from build123d import *

# Parameters (mm, degrees)
SKETCH2_R           = 88.9
BOSS_EXTRUDE1_DEPTH = 3.175
SKETCH3_R           = 3.175
SKETCH3_W           = 50.8
SKETCH3_H           = 71.12
CUT_EXTRUDE1_DEPTH  = 3.175
SKETCH5_W           = 3
SKETCH5_H           = 3
SKETCH5_R           = 3.175
CUT_EXTRUDE2_DEPTH  = 126.763669734
FILLET1_R           = 22.86
SKETCH6_R           = 6.35
CUT_EXTRUDE3_DEPTH  = 126.763669734


with BuildPart() as part:
    # Sketch2 → Boss-Extrude1 (new body)
    with BuildSketch(Plane(origin=(0, 0, 0), x_dir=(1, 0, 0), z_dir=(0, 1, 0))):
        with Locations(Location((0, 0, 0), (0, 0, 270))):
            Circle(SKETCH2_R)
    extrude(amount=BOSS_EXTRUDE1_DEPTH)

    # Sketch3 → Cut-Extrude1 (cut)
    with BuildSketch(Plane(origin=(0, 3.175, 0), x_dir=(1, 0, 0), z_dir=(0, 1, 0))):
        with Locations(Location((65.549718535, -24.13, 0), (0, 0, 270))):
            Circle(SKETCH3_R)
        with Locations(Location((65.549718535, 24.13, 0), (0, 0, 270))):
            Circle(SKETCH3_R)
        with Locations(Location((-53.672052261, 44.702721462, 0), (0, 0, 270))):
            Circle(SKETCH3_R)
        with Locations(Location((-11.877666274, 68.832721462, 0), (0, 0, 270))):
            Circle(SKETCH3_R)
        with Locations(Location((-11.877666274, -68.832721462, 0), (0, 0, 270))):
            Circle(SKETCH3_R)
        with Locations(Location((-53.672052261, -44.702721462, 0), (0, 0, 270))):
            Circle(SKETCH3_R)
        with Locations((-63.5, 0)):
            Rectangle(SKETCH3_W, SKETCH3_H)
    extrude(amount=-CUT_EXTRUDE1_DEPTH, mode=Mode.SUBTRACT)

    # Sketch5 → Cut-Extrude2 (cut, through all)
    with BuildSketch(Plane(origin=(0, 3.175, 0), x_dir=(1, 0, 0), z_dir=(0, 1, 0))):
        with Locations((-36.6, 57.12)):
            Rectangle(SKETCH5_W, SKETCH5_H)
        with Locations((-28.98, 1.04)):
            Rectangle(SKETCH5_W, SKETCH5_H)
        with Locations(Location((61.9, 44.62, 0), (0, 0, 270))):
            Circle(SKETCH5_R)
        with Locations(Location((47.695, -21.96, 0), (0, 0, 270))):
            Circle(SKETCH5_R)
    extrude(amount=-CUT_EXTRUDE2_DEPTH, mode=Mode.SUBTRACT)

    # Fillet1
    fillet1_edges = [part.edges().sort_by_distance(p)[0] for p in [
        (-38.1, 1.5875, 35.56),
        (-38.1, 1.5875, -35.56),
    ]]
    fillet(fillet1_edges, radius=FILLET1_R)

    # Sketch6 → Cut-Extrude3 (cut, through all)
    with BuildSketch(Plane(origin=(0, 3.175, 0), x_dir=(1, 0, 0), z_dir=(0, 1, 0))):
        with Locations(Location((65.549718535, 0, 0), (0, 0, 270))):
            Circle(SKETCH6_R)
        with BuildLine():
            Line((8.442333726, 75.182721462), (33.842333726, 75.182721462))
            ThreePointArc((33.842333726, 75.182721462), (40.192333726, 68.832721462), (33.842333726, 62.482721462))
            Line((33.842333726, 62.482721462), (8.442333726, 62.482721462))
            ThreePointArc((8.442333726, 62.482721462), (2.092333726, 68.832721462), (8.442333726, 75.182721462))
        make_face()
        with BuildLine():
            Line((8.442333726, -62.482721462), (33.842333726, -62.482721462))
            ThreePointArc((33.842333726, -62.482721462), (40.192333726, -68.832721462), (33.842333726, -75.182721462))
            Line((33.842333726, -75.182721462), (8.442333726, -75.182721462))
            ThreePointArc((8.442333726, -75.182721462), (2.092333726, -68.832721462), (8.442333726, -62.482721462))
        make_face()
    extrude(amount=-CUT_EXTRUDE3_DEPTH, mode=Mode.SUBTRACT)


solid = part.part
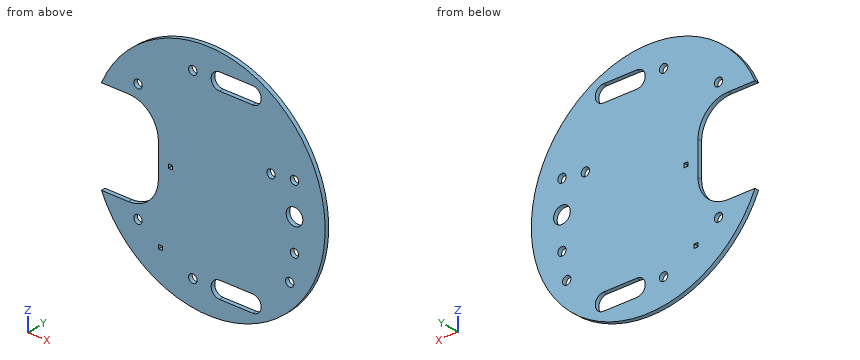
Geometry check sheet. Reference: the model listing, model coordinates, mm. Give positions to 0.01 mm unless a question says otherwise; leave off trailing zeros. Loops run counter-clockwise (first coordinate to the right, second up) from the corner with the lowest first, then second, coordinate; pieces in that order, holes last.
(1) Thickness scan on L1, parallel to X at y = 1.45, z = 24.13; L2, parallel to X at y = 1.6, z = -44.62 (3 decimals); L3, parallel to X at y = 1, z = -4. Record the ranges inside material, lowest first.
From the geometry:
L1: x = -41.16 to 45.38, 50.01 to 62.37, 68.72 to 85.56
L2: x = -76.891 to -56.846, -50.498 to 58.725, 65.075 to 76.891
L3: x = -38.1 to 60.62, 70.48 to 88.81
(2) Section check A-A on z = -44.62. Record the cut outline in (x, y) (3 decimals), then the cut area to 3 significant figures.
From the geometry:
outline: (-76.891, 0) - (-56.846, 0) - (-56.846, 3.175) - (-76.891, 3.175) - close; (-50.498, 0) - (58.725, 0) - (58.725, 3.175) - (-50.498, 3.175) - close; (65.075, 0) - (76.891, 0) - (76.891, 3.175) - (65.075, 3.175) - close
area: 448 mm2
(3) Depth check by flat-ended pin: pin 1 Ø1.5 at (x, y) = (-37, 2) entering from -Z; pin 2 Ø8.5 at (x, z) = (65.55, -24.13) entering from -Y; pin 3 Ø1 at (y, z) = (0.5, 7.5) entering from -X; pin 4 Ø5.5 at (x, z) = (-53.67, 44.7) entering from +Y. Enter the tip coordinate at first touch or a pass-through.
From the geometry:
pin 1: stops at z = -81.17
pin 2: stops at y = 0
pin 3: stops at x = -38.1
pin 4: passes through
(4) Section check C-C on y = 1.65. Count the separate pieces of the cut face and the enclosed holes in it, then the cut area to 3 significant figures.
From the geometry:
separate pieces: 1
enclosed holes: 13
area: 20,300 mm2
(5) Section check D-D on z = 30.5. Record the cut outline in (x, y) (3 decimals).
From the geometry:
outline: (-46.616, 0) - (83.504, 0) - (83.504, 3.175) - (-46.616, 3.175) - close
(6) Section check B-B on x = -41.5. Record the cut outline in (y, z) (3 decimals).
From the geometry:
outline: (0, -78.619) - (3.175, -78.619) - (3.175, -24.695) - (0, -24.695) - close; (0, 24.695) - (3.175, 24.695) - (3.175, 78.619) - (0, 78.619) - close
